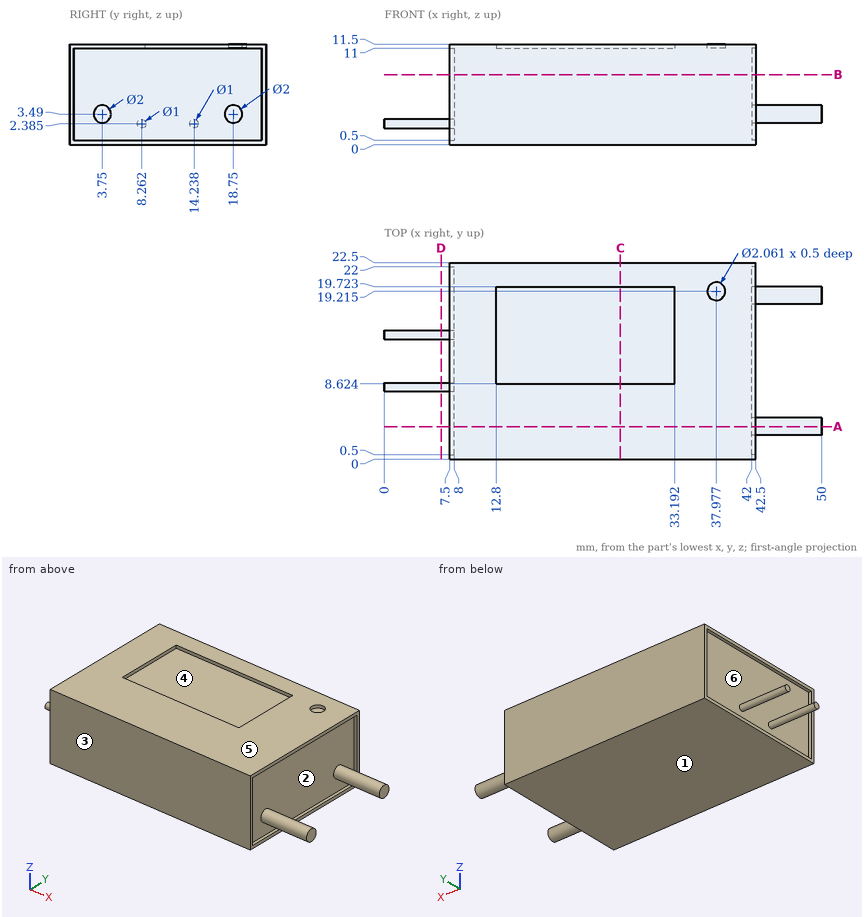
Geometry check sheet. Reference: drawing and pictorial views, mm from the part's lowest x, y, z. A direction names the side the tool comes from. Give positions to 0.01 mm unless a question says otherwise; leave off trailing zeros. Order: outer loops, then holes, each group sorted by start corner. A loop starts at its lowest first (then second) coordinate and runs counter-clockwise, first axis right, second up. Notation, with made-up numbers: (-9.5, -34) -> (19.5, -34) arc R20 ccw to (19.5, -27) -> close; hole circle Ø3 at (-8.5, 24.25). An arc over 180 degrees is marked (long way). Write each question's results on one line, items separated by ' | '. Start each with the question number.
(1) Sectioned sample at C-C (x = 27). Enter the section's corners in (y, z), plus the area to 3 significant figures.
(2) Mould release check, pull along Z, two halves, no side actions. Record for the marked faces 1, 2 and 3: pulls with the +Z half, pulls with the -Z half, needs draft (parallel to the pull), parting line crosses it, or undercut.
(3) Sectioned sample at A-A (y = 3.75). Enter the section's corners in (x, z), plus the area to 3 significant figures.
(4) Access from +Z, -Z, +X, -X, +Y, -Y to the whole of each face (thin tool, end or side, straight path). Record for the marked faces 4, 5 and 6.
(5) Sectioned sample at D-D (x = 6.5). Enter the section's corners in (y, z) (1 decimal).
(6) Scan lines: line 1 (X direction, y = 5.5, z = 4); line 2 (Z direction, x = 13, y = 16.5); line 3 (Z direction, x = 46, y = 3). Record each from-to range of solid material in increasing order.
(7) Gauge pin test, flat ends, axial feed: P1, Ø9, axis at x = 22, y = 15, coming from the +Z side; P2, Ø0.6, axis at y = 15.5, z = 11, coming from the +X side. Record the tip position at first contact, or that the pin passes through.
(8) Sectioned sample at B-B (z = 8). Enter the section's corners in (x, y), plus the area to 3 significant figures.
Answer below:
1) outline: (0, 0) -> (22.5, 0) -> (22.5, 11.5) -> (19.72, 11.5) -> (19.72, 11) -> (8.62, 11) -> (8.62, 11.5) -> (0, 11.5) -> close | area: 253 mm2
2) face 1: pulls with the -Z half | face 2: undercut | face 3: needs draft
3) outline: (7.5, 0) -> (42.5, 0) -> (42.5, 0.5) -> (42, 0.5) -> (42, 2.49) -> (50, 2.49) -> (50, 4.49) -> (42, 4.49) -> (42, 11) -> (42.5, 11) -> (42.5, 11.5) -> (7.5, 11.5) -> (7.5, 11) -> (8, 11) -> (8, 0.5) -> (7.5, 0.5) -> close | area: 408 mm2
4) face 4: +Z | face 5: +Z, +X, -X, +Y, -Y | face 6: -X
5) outline: circle Ø1 at (8.3, 2.4); circle Ø1 at (14.2, 2.4)
6) line 1: 8 to 42 | line 2: 0 to 11 | line 3: 2.83 to 4.15
7) P1: z = 11 | P2: x = 42.5
8) outline: (7.5, 0) -> (42.5, 0) -> (42.5, 0.5) -> (42, 0.5) -> (42, 22) -> (42.5, 22) -> (42.5, 22.5) -> (7.5, 22.5) -> (7.5, 22) -> (8, 22) -> (8, 0.5) -> (7.5, 0.5) -> close | area: 766 mm2
